Autodesk Inventor part; units mm, degrees
ref_plane "YZ Plane" through (0, 0, 0) normal (1, 0, 0) x (0, 1, 0)
ref_plane "XZ Plane" through (0, 0, 0) normal (0, 1, 0) x (-1, 0, 0)
ref_plane "XY Plane" through (0, 0, 0) normal (0, 0, 1) x (1, 0, 0)
sketch "Skizze1" plane through (0, 0, 0) normal (0, 1, 0) x (-1, 0, 0)
  line L0 (-20, 20) -> (20, 20)
  line L1 (20, 20) -> (20, -20)
  line L2 (20, -20) -> (-20, -20)
  line L3 (-20, -20) -> (-20, 20)
  line L4 (-20, 20) -> (20, -20) construction
  line L5 (20, 20) -> (-20, -20) construction
  line L6 (20, 20) -> (0, 20) construction
  line L7 (0, 20) -> (0, 0) construction
  line L8 (0, 0) -> (20, 0) construction
  line L9 (20, 0) -> (20, 20) construction
  line L10 (0, 0) -> (-20, 0) construction
  line L11 (-20, 0) -> (-20, -20) construction
  line L12 (-20, -20) -> (0, -20) construction
  line L13 (0, -20) -> (0, 0) construction
  point P0 (10, 10)
  point P1 (-10, -10)
  dimension "d0" = 40
  dimension "d1" = 40
extrude "Extrusion1" add sketch "Skizze1" along normal blind 3
sketch "Skizze2" plane through (0, 0, 0) normal (0, -1, 0) x (1, 0, 0)
  line L0 (20, -20) -> (-20, -20) construction
  line L1 (20, 20) -> (20, -20) construction
  line L2 (-20, 20) -> (20, 20) construction
  line L3 (-20, -20) -> (-20, 20) construction
  line L4 (20, 20) -> (0, 20) construction
  line L5 (0, 20) -> (0, 0) construction
  line L6 (0, 0) -> (20, 0) construction
  line L7 (20, 0) -> (20, 20) construction
  line L8 (-20, -20) -> (0, -20) construction
  line L9 (0, -20) -> (0, 0) construction
  line L10 (0, 0) -> (-20, 0) construction
  line L11 (-20, 0) -> (-20, -20) construction
  circle A0 centre (10, 10) radius 5.25
  circle A1 centre (-10, -10) radius 5.25
  dimension "d4" = 10.5
  dimension "d5" = 10.5
extrude "Extrusion2" cut sketch "Skizze2" against normal blind 2
sketch "Skizze4" plane through (0, 0, 0) normal (0, -1, 0) x (1, 0, 0)
  line L0 (20, 20) -> (20, -20)
  line L1 (-20, -20) -> (-20, 20)
  line L2 (-20, 20) -> (20, 20)
  line L3 (20, -20) -> (-20, -20)
  line L4 (20, 20) -> (-20, 20)
  line L5 (-20, 20) -> (-20, -20)
  line L6 (-20, -20) -> (20, -20)
  line L7 (20, -20) -> (20, 20)
  point P0 (0, 0)
extrude "Extrusion3" add sketch "Skizze4" along normal blind 47
sketch "Sketch6" plane through (0, -47, 0) normal (0, -1, 0) x (1, 0, 0)
  circle A0 centre (0, 0) radius 2
  dimension "d20" = 4
extrude "Extrusion4" cut sketch "Sketch6" against normal blind 6
fillet "Fillet1" radius 5 4 edges at (-20, -22, 20) (-20, -22, -20) (20, -22, -20) (20, -22, 20)
ref_plane "Arbeitsebene2" through (-18.5355, -47, -18.5355) normal (-0.7071, 0, 0.7071) x (0.7071, 0, 0.7071)
properties part number "Stützblöcke"
Verification items for the finished model (mm, model axes). A direction names the side the tool comes from. Round coordinates to 2 decimals unless told otherwise and drop trailing zeros. Loops run counter-clockwise (first coordinate to the right, second up) from the corner with the lowest first, then second, coordinate; pieces in that order, holes last. Notation, with made-up numbers: (24.5, 63) - (63.5, 63) arc R27 cw to (63.5, 91) - close; hole circle Ø1 at (-7.5, -10.75). An arc over 180 degrees is marked (long way). Use a Markdown table: item, result. Add a question column.
1. Thickness scan on probe 1 along Y at (x, z) = (9, 13); probe 2 along Z at (x, y) = (10, 1); probe 3 along X at (y, z) = (-16, 18). Record the ranges inside material, lowest first. Write a range as [from, to].
2. Access from +Z, -Z, +X, -X, +Y, -Y to the whole of each face (thin tool, end or side, straight path). Record for faces 1 (the face through (0, -22, 20)), 2 (the face through (0, -44, -2)), 3 (the face through (10, 2, 10)).
3. Section check A-A, the plane x = -17. Record the boundary of the cut face in (y, z), plus the area to 3 significant figures.
4. Release check for a two-part mould opening along Y. For faces 4 (the face through (20, -22, 0)), 5 (the face through (-10, 0, -10)), 6 (the face through (0, 3, 0)) record: released by +Y, released by -Y, zero draft, split by the parting line, or undercut.
5. Gauge pin test, flat end, axial feed: pin 1 (3 mm diameter, centred on x = 0, z = 0, fed in from -Y). Record the tip position at first contact, or that the pin passes through.
Checks:
| question | item | result |
|---|---|---|
| 1 | probe 1 | y = [-47, 0], [2, 3] |
| 1 | probe 2 | z = [-20, 4.75], [15.25, 20] |
| 1 | probe 3 | x = [-19, 19] |
| 2 | face 1 | +Z, +X, -X, +Y, -Y |
| 2 | face 2 | -Y |
| 2 | face 3 | none |
| 3 | outline | (-47, -19.58) - (3, -19.58) - (3, 19.58) - (-47, 19.58) - close |
| 3 | area | 1,960 mm^2 |
| 4 | face 4 | zero draft |
| 4 | face 5 | undercut |
| 4 | face 6 | released by +Y |
| 5 | pin 1 | stops at y = -41 |
